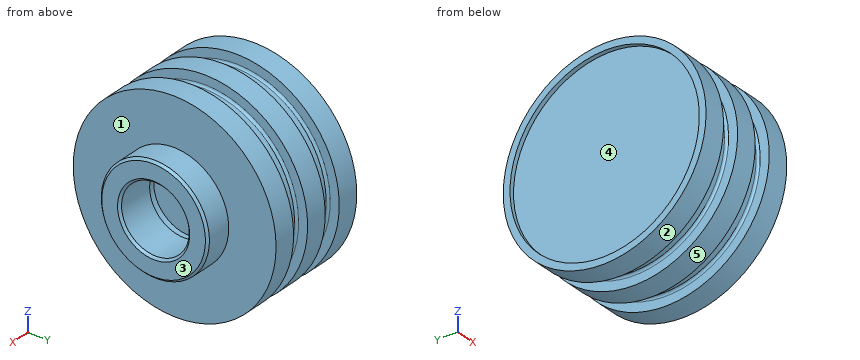
from build123d import *

# Parameters (mm, degrees)
CHAMFER_1_SIZE = 1


with BuildPart() as part:
    # Эскиз1 → Повернуть1 (revolve)
    with BuildSketch(Plane.XY, mode=Mode.PRIVATE) as revolve_1_sk:
        with BuildLine():
            Line((0, 42), (0, 45))
            Line((0, 45), (10, 45))
            Line((10, 45), (10, 41))
            ThreePointArc((10, 41), (10.292893219, 40.292893219), (11, 40))
            Line((11, 40), (17, 40))
            ThreePointArc((17, 40), (17.707106781, 40.292893219), (18, 41))
            Line((18, 41), (18, 45))
            Line((18, 45), (28, 45))
            Line((28, 45), (28, 41))
            ThreePointArc((28, 41), (28.292893219, 40.292893219), (29, 40))
            Line((29, 40), (35, 40))
            ThreePointArc((35, 40), (35.707106781, 40.292893219), (36, 41))
            Line((36, 41), (36, 45))
            Line((36, 45), (46, 45))
            Line((46, 45), (46, 24))
            Line((46, 24), (57, 24))
            Line((57, 24), (58, 23))
            Line((58, 23), (58, 0))
            Line((58, 0), (2, 0))
            Line((2, 0), (2, 42))
            Line((2, 42), (0, 42))
        make_face()
    revolve(revolve_1_sk.sketch.rotate(Axis((2, 0, 0), (1, 0, 0)), 90), axis=Axis((2, 0, 0), (1, 0, 0)))

    # Эскиз2 → Вырез-Повернуть1 (revolve, cut)
    with BuildSketch(Plane.XY, mode=Mode.PRIVATE) as cut_revolve_1_sk:
        Polygon((58, 0), (58, 15), (41, 15), (41, 15.5), (38, 15.5), (38, 0), align=None)
    revolve(cut_revolve_1_sk.sketch.rotate(Axis((0, 0, 0), (1, 0, 0)), 90), axis=Axis((0, 0, 0), (1, 0, 0)), mode=Mode.SUBTRACT)

    # Фаска1
    chamfer_1_edges = [part.edges().sort_by_distance(p)[0] for p in [
        (58, 0, -15),
    ]]
    chamfer(chamfer_1_edges, length=CHAMFER_1_SIZE)


solid = part.part
Verification items for the finished model (mm, model axes). Face numbers are marked on the shaded views. A direction names the side the tool comes from. Give positions to 0.01 mm unless a question says otherwise; leave off trailing zeros. Loops run counter-clockwise (first coordinate to the right, second up) from the corner with the lowest first, then second, coordinate; pieces in that order, holes last.
1) Set-up check for the marked faces 1 and 2: record each of +Z, -Z, +X, -X, +Y, -Y from which the full face is reachable in a straight line by a thin tool's end or side.
2) Sectioned sample at C-C, the plane x = 43. Enter the section's corners in (y, z).
3) Depth check by flat-ended pin: pin 1 Ø5 at (x, y) = (32, -25.5) entering from -Z; pin 2 Ø25 at (y, z) = (-2.5, 3.5) entering from -X; pin 3 Ø5 at (y, z) = (-30.5, 22.5) entering from +X. Enter the tip coordinate at first touch or a pass-through.
4) Sectioned sample at A-A, the plane x = 49. Enter the section's corners in (y, z).
5) Thickness scan on line 1 along Y through (x, z) = (53, 0); line 2 along X through (y, z) = (-19, 25); line 3 along Y through (x, z) = (1, 0). Record the ranges inside material, lowest first.
6) Draft check along Z on the marked faces 3, 4 and 5. Enter one of: pulls with the +Z half, pulls with the -Z half, needs draft (parallel to the pull), parting line crosses it, or undercut.
7) Sectioned sample at B-B, the plane x = 33.5. Enter the section's corners in (y, z), then the cut area to 3 significant figures.
Answers:
1. face 1: +X
1. face 2: +X, -X
2. outline: circle Ø90 at (0, 0); hole circle Ø30 at (0, 0)
3. pin 1: stops at z = -32.73
3. pin 2: stops at x = 2
3. pin 3: stops at x = 46
4. outline: circle Ø48 at (0, 0); hole circle Ø30 at (0, 0)
5. line 1: y = -24 to -15, 15 to 24
5. line 2: x = 2 to 46
5. line 3: y = -45 to -42, 42 to 45
6. face 3: needs draft
6. face 4: undercut
6. face 5: parting line crosses it
7. outline: circle Ø80 at (0, 0)
7. area: 5,030 mm2
